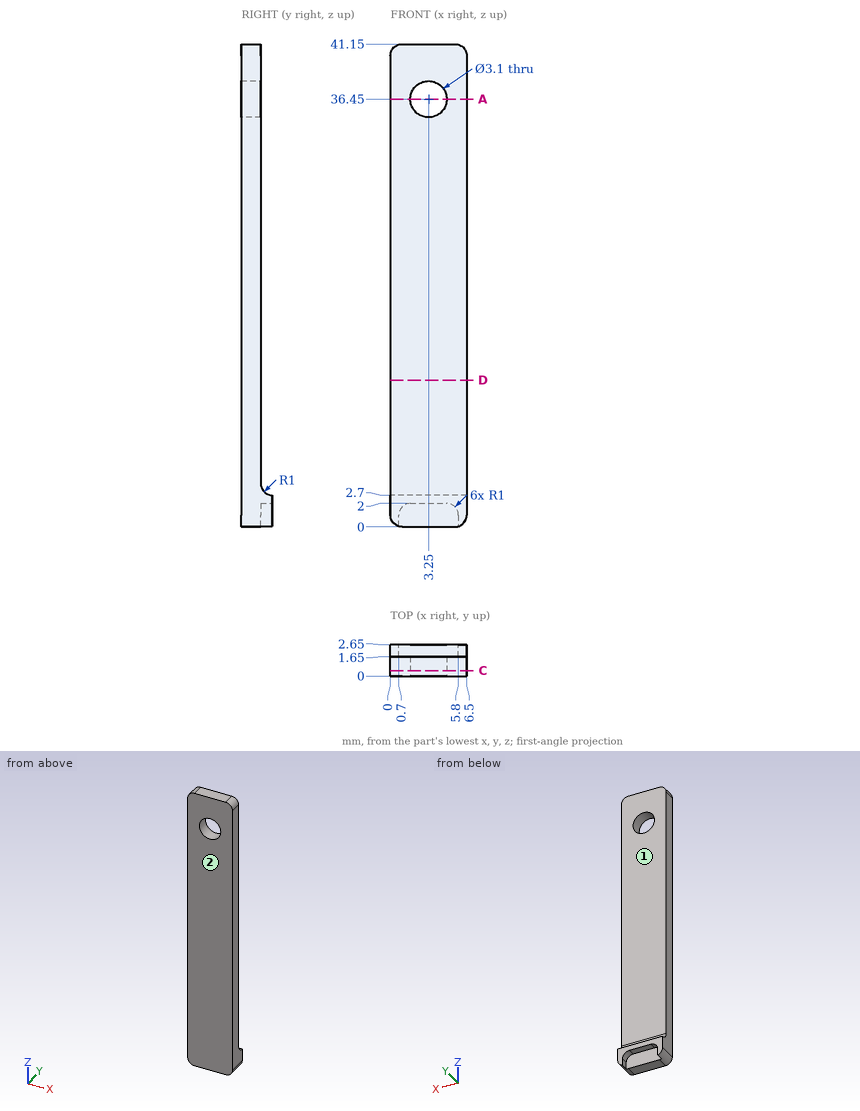
Could you check a few things on this drawing? It's one solid part, dimensions in mm from its lowest x, y, z. A direction names the side the tool comes from. Round coordinates to 2 decimals unless told otherwise and drop trailing zeros. Loops run counter-clockwise (first coordinate to the right, second up) from the corner with the lowest first, then second, coordinate; pieces in that order, holes last. Notation, with made-up numbers: (-26.5, 31.25) -> (-14.5, 31.25) arc R19 ccw to (-14.5, 46.25) -> close; hole circle Ø9 at (59.25, -10). An arc over 180 degrees is marked (long way). Answer as CSV lines item,"result".
1. If we section it at D-D on z = 12.5: Please give me the cut outline in (x, y).
Final values:
outline,"(0, 0) -> (6.5, 0) -> (6.5, 1.65) -> (0, 1.65) -> close"
2. For pin 1 (3 mm diameter, centred on x = 4, z = 6, fed in from +Y); pin 2 (1.9 mm diameter, centred on x = 3.25, z = 36.45, fed in from +Y), each with a flat end and sliding along its axis, tell me the tip position at first contact or that it passes through.
Final values:
pin 1,"stops at y = 1.65"
pin 2,"passes through"
3. If I drill on L1, parallel to X at y = 0.65, z = 36.45; L2, parallel to Y at x = 0.5, z = 23; L3, parallel to Z at x = 3.5, y = 0.9, over which ranges is the centre line in solid material (lowest first)?
Final values:
L1,"x = 0 to 1.7, 4.8 to 6.5"
L2,"y = 0 to 1.65"
L3,"z = 0 to 34.92, 37.98 to 41.15"
4. If we section it at A-A on z = 36.45: Please give me the cut outline in (x, y), plus the area to 3 significant figures.
Final values:
outline,"(0, 0) -> (1.7, 0) -> (1.7, 1.65) -> (0, 1.65) -> close; (4.8, 0) -> (6.5, 0) -> (6.5, 1.65) -> (4.8, 1.65) -> close"
area,"5.61 mm^2"
5. Which directions (+Z, -Z, +X, -X, +Y, -Y) give clear straight access to the entire face, cutting with the end or side of a thin tool? Please do the marked faces 1 and 2.
Final values:
face 1,"+Z, +X, -X, +Y"
face 2,"+Z, -Z, +X, -X, -Y"
6. If we section it at C-C on y = 0.45: Please give me the cut outline in (x, z), plus the area to 3 significant figures.
Final values:
outline,"(0, 1) arc R1 ccw to (1, 0) -> (5.5, 0) arc R1 ccw to (6.5, 1) -> (6.5, 40.15) arc R1 ccw to (5.5, 41.15) -> (1, 41.15) arc R1 ccw to (0, 40.15) -> close; hole circle Ø3.1 at (3.25, 36.45)"
area,"259 mm^2"
